Autodesk Inventor part; units mm, degrees
ref_plane "YZ Plane" through (0, 0, 0) normal (1, 0, 0) x (0, 1, 0)
ref_plane "XZ Plane" through (0, 0, 0) normal (0, 1, 0) x (-1, 0, 0)
ref_plane "XY Plane" through (0, 0, 0) normal (0, 0, 1) x (1, 0, 0)
sketch "草图1" plane through (0, 0, 0) normal (0, 0, 1) x (1, 0, 0)
  circle A0 centre (0, 0) radius 12.5
  dimension "d0" = 25
extrude "拉伸1" add sketch "草图1" along normal blind 40
sketch "草图2" plane through (0, 0, 40) normal (0, 0, 1) x (1, 0, 0)
  circle A0 centre (0, 0) radius 20
  point P0 (0, 0)
extrude "拉伸2" add sketch "草图2" along normal blind 250
sketch "草图3" plane through (0, 0, 290) normal (0, 0, 1) x (1, 0, 0)
  circle A0 centre (0, 0) radius 10
  dimension "d5" = 20
extrude "拉伸3" add sketch "草图3" along normal blind 40
properties part number "传动轴2"
Geometry check sheet. Reference: the model listing, model coordinates, mm. A direction names the side the tool comes from. Give positions to 0.01 mm unless a question says otherwise; leave off trailing zeros. Loops run counter-clockwise (first coordinate to the right, second up) from the corner with the lowest first, then second, coordinate; pieces in that order, holes last. Notation, with made-up numbers: M 22,-39 L 43,-39 A17 ccw 43,-26 Z; hole C 65.25,45.5 d4. An arc over 180 degrees is marked long. Write each question's results on one line, items separated by ' | '.
1) Section check D-D, the plane y = 17. Record the boundary of the cut face in (x, z), plus the area to 3 significant figures.
Answers follow:
outline: M -10.54,40 L 10.54,40 L 10.54,290 L -10.54,290 Z | area: 5,270 mm2
2) Section check C-C, the plane z = 54.5. Record the boundary of the cut face in (x, y).
Answers follow:
outline: C 0,0 d40
3) Gauge pin test, flat ends, axial feed: pin 1 (4 mm diameter, centred on y = 7, z = 52, fed in from +X); pin 2 (10 mm diameter, centred on x = -2.5, y = -12, fed in from -Z); pin 3 (1.5 mm diameter, centred on y = -3.5, z = 199, fed in from +X); pin 4 (2 mm diameter, centred on y = 5, z = 251.5, fed in from -X). Record the tip position at first contact, or that the pin passes through.
Answers follow:
pin 1: x = 19.36 | pin 2: z = 0 | pin 3: x = 19.81 | pin 4: x = -19.6
4) Thickness scan on line 1 (Y direction, x = 0, z = 262); line 2 (Z direction, x = 5.5, y = 13.5); line 3 (Z direction, x = -8, y = 8.5). Record the ranges inside material, lowest first.
Answers follow:
line 1: -20 to 20 | line 2: 40 to 290 | line 3: 0 to 290
5) Section check A-A, the plane y = 0. Record the boundary of the cut face in (x, z), plus the area to 3 significant figures.
Answers follow:
outline: M -20,40 L -12.5,40 L -12.5,0 L 12.5,0 L 12.5,40 L 20,40 L 20,290 L 10,290 L 10,330 L -10,330 L -10,290 L -20,290 Z | area: 11,800 mm2
6) Tool access check on faces 1 (the face through (9, 9, 40)), 2 (the face through (-2.17, 9.76, 309.72)), 3 (the face through (0, 0, 0)). Record the directions out of +Z, -Z, +X, -X, +Y, -Y that give a thin tool (end or side, any length) a straight path to the whole face; none if there is none.
Answers follow:
face 1: -Z | face 2: +Z | face 3: -Z, +X, -X, +Y, -Y
